```python
from build123d import *

# Parameters (mm, degrees)
SKETCH3_R           = 3.5
BOSS_EXTRUDE1_DEPTH = 304.8


with BuildPart() as part:
    # Sketch3 → Boss-Extrude1 (new, symmetric)
    with BuildSketch(Plane.XY):
        with BuildLine():
            Line((15.25, 20), (-15.25, 20))
            ThreePointArc((-15.25, 20), (-15.780330086, 19.780330086), (-16, 19.25))
            Line((-16, 19.25), (-16, 16.25))
            ThreePointArc((-16, 16.25), (-15.780330086, 15.719669914), (-15.25, 15.5))
            Line((-15.25, 15.5), (-9.931980515, 15.5))
            ThreePointArc((-9.931980515, 15.5), (-9.070942793, 14.924672987), (-9.272970773, 13.909009742))
            Line((-9.272970773, 13.909009742), (-15.140128061, 8.041852455))
            ThreePointArc((-15.140128061, 8.041852455), (-15.740311256, 7.640822865), (-16.448275606, 7.5))
            Line((-16.448275606, 7.5), (-23.551724394, 7.5))
            ThreePointArc((-23.551724394, 7.5), (-24.259688744, 7.640822865), (-24.859871939, 8.041852455))
            Line((-24.859871939, 8.041852455), (-30.727029227, 13.909009742))
            ThreePointArc((-30.727029227, 13.909009742), (-30.929057207, 14.924672987), (-30.068019485, 15.5))
            Line((-30.068019485, 15.5), (-24.75, 15.5))
            ThreePointArc((-24.75, 15.5), (-24.219669914, 15.719669914), (-24, 16.25))
            Line((-24, 16.25), (-24, 19.25))
            ThreePointArc((-24, 19.25), (-24.219669914, 19.780330086), (-24.75, 20))
            Line((-24.75, 20), (-37, 20))
            ThreePointArc((-37, 20), (-39.121320344, 19.121320344), (-40, 17))
            Line((-40, 17), (-40, 4.75))
            ThreePointArc((-40, 4.75), (-39.780330086, 4.219669914), (-39.25, 4))
            Line((-39.25, 4), (-36.25, 4))
            ThreePointArc((-36.25, 4), (-35.719669914, 4.219669914), (-35.5, 4.75))
            Line((-35.5, 4.75), (-35.5, 10.068019485))
            ThreePointArc((-35.5, 10.068019485), (-34.924672987, 10.929057207), (-33.909009742, 10.727029227))
            Line((-33.909009742, 10.727029227), (-28.041852455, 4.859871939))
            ThreePointArc((-28.041852455, 4.859871939), (-27.640822865, 4.259688744), (-27.5, 3.551724394))
            Line((-27.5, 3.551724394), (-27.5, -3.551724394))
            ThreePointArc((-27.5, -3.551724394), (-27.640822865, -4.259688744), (-28.041852455, -4.859871939))
            Line((-28.041852455, -4.859871939), (-33.909009742, -10.727029227))
            ThreePointArc((-33.909009742, -10.727029227), (-34.924672987, -10.929057207), (-35.5, -10.068019485))
            Line((-35.5, -10.068019485), (-35.5, -4.75))
            ThreePointArc((-35.5, -4.75), (-35.719669914, -4.219669914), (-36.25, -4))
            Line((-36.25, -4), (-39.25, -4))
            ThreePointArc((-39.25, -4), (-39.780330086, -4.219669914), (-40, -4.75))
            Line((-40, -4.75), (-40, -17))
            ThreePointArc((-40, -17), (-39.121320344, -19.121320344), (-37, -20))
            Line((-37, -20), (-24.75, -20))
            ThreePointArc((-24.75, -20), (-24.219669914, -19.780330086), (-24, -19.25))
            Line((-24, -19.25), (-24, -16.25))
            ThreePointArc((-24, -16.25), (-24.219669914, -15.719669914), (-24.75, -15.5))
            Line((-24.75, -15.5), (-30.068019485, -15.5))
            ThreePointArc((-30.068019485, -15.5), (-30.929057207, -14.924672987), (-30.727029227, -13.909009742))
            Line((-30.727029227, -13.909009742), (-24.859871939, -8.041852455))
            ThreePointArc((-24.859871939, -8.041852455), (-24.259688744, -7.640822865), (-23.551724394, -7.5))
            Line((-23.551724394, -7.5), (-16.448275606, -7.5))
            ThreePointArc((-16.448275606, -7.5), (-15.740311256, -7.640822865), (-15.140128061, -8.041852455))
            Line((-15.140128061, -8.041852455), (-9.272970773, -13.909009742))
            ThreePointArc((-9.272970773, -13.909009742), (-9.070942793, -14.924672987), (-9.931980515, -15.5))
            Line((-9.931980515, -15.5), (-15.25, -15.5))
            ThreePointArc((-15.25, -15.5), (-15.780330086, -15.719669914), (-16, -16.25))
            Line((-16, -16.25), (-16, -19.25))
            ThreePointArc((-16, -19.25), (-15.780330086, -19.780330086), (-15.25, -20))
            Line((-15.25, -20), (15.25, -20))
            ThreePointArc((15.25, -20), (15.780330086, -19.780330086), (16, -19.25))
            Line((16, -19.25), (16, -16.25))
            ThreePointArc((16, -16.25), (15.780330086, -15.719669914), (15.25, -15.5))
            Line((15.25, -15.5), (9.931980515, -15.5))
            ThreePointArc((9.931980515, -15.5), (9.070942793, -14.924672987), (9.272970773, -13.909009742))
            Line((9.272970773, -13.909009742), (15.140128061, -8.041852455))
            ThreePointArc((15.140128061, -8.041852455), (15.740311256, -7.640822865), (16.448275606, -7.5))
            Line((16.448275606, -7.5), (23.551724394, -7.5))
            ThreePointArc((23.551724394, -7.5), (24.259688744, -7.640822865), (24.859871939, -8.041852455))
            Line((24.859871939, -8.041852455), (30.727029227, -13.909009742))
            ThreePointArc((30.727029227, -13.909009742), (30.929057207, -14.924672987), (30.068019485, -15.5))
            Line((30.068019485, -15.5), (24.75, -15.5))
            ThreePointArc((24.75, -15.5), (24.219669914, -15.719669914), (24, -16.25))
            Line((24, -16.25), (24, -19.25))
            ThreePointArc((24, -19.25), (24.219669914, -19.780330086), (24.75, -20))
            Line((24.75, -20), (37, -20))
            ThreePointArc((37, -20), (39.121320344, -19.121320344), (40, -17))
            Line((40, -17), (40, -4.75))
            ThreePointArc((40, -4.75), (39.780330086, -4.219669914), (39.25, -4))
            Line((39.25, -4), (36.25, -4))
            ThreePointArc((36.25, -4), (35.719669914, -4.219669914), (35.5, -4.75))
            Line((35.5, -4.75), (35.5, -10.068019485))
            ThreePointArc((35.5, -10.068019485), (34.924672987, -10.929057207), (33.909009742, -10.727029227))
            Line((33.909009742, -10.727029227), (28.041852455, -4.859871939))
            ThreePointArc((28.041852455, -4.859871939), (27.640822865, -4.259688744), (27.5, -3.551724394))
            Line((27.5, -3.551724394), (27.5, 3.551724394))
            ThreePointArc((27.5, 3.551724394), (27.640822865, 4.259688744), (28.041852455, 4.859871939))
            Line((28.041852455, 4.859871939), (33.909009742, 10.727029227))
            ThreePointArc((33.909009742, 10.727029227), (34.924672987, 10.929057207), (35.5, 10.068019485))
            Line((35.5, 10.068019485), (35.5, 4.75))
            ThreePointArc((35.5, 4.75), (35.719669914, 4.219669914), (36.25, 4))
            Line((36.25, 4), (39.25, 4))
            ThreePointArc((39.25, 4), (39.780330086, 4.219669914), (40, 4.75))
            Line((40, 4.75), (40, 17))
            ThreePointArc((40, 17), (39.121320344, 19.121320344), (37, 20))
            Line((37, 20), (24.75, 20))
            ThreePointArc((24.75, 20), (24.219669914, 19.780330086), (24, 19.25))
            Line((24, 19.25), (24, 16.25))
            ThreePointArc((24, 16.25), (24.219669914, 15.719669914), (24.75, 15.5))
            Line((24.75, 15.5), (30.068019485, 15.5))
            ThreePointArc((30.068019485, 15.5), (30.929057207, 14.924672987), (30.727029227, 13.909009742))
            Line((30.727029227, 13.909009742), (24.859871939, 8.041852455))
            ThreePointArc((24.859871939, 8.041852455), (24.259688744, 7.640822865), (23.551724394, 7.5))
            Line((23.551724394, 7.5), (16.448275606, 7.5))
            ThreePointArc((16.448275606, 7.5), (15.740311256, 7.640822865), (15.140128061, 8.041852455))
            Line((15.140128061, 8.041852455), (9.272970773, 13.909009742))
            ThreePointArc((9.272970773, 13.909009742), (9.070942793, 14.924672987), (9.931980515, 15.5))
            Line((9.931980515, 15.5), (15.25, 15.5))
            ThreePointArc((15.25, 15.5), (15.780330086, 15.719669914), (16, 16.25))
            Line((16, 16.25), (16, 19.25))
            ThreePointArc((16, 19.25), (15.780330086, 19.780330086), (15.25, 20))
        make_face()
        with Locations(Location((-20, 0, 0), (0, 0, 180))):
            Circle(SKETCH3_R, mode=Mode.SUBTRACT)
        with Locations(Location((20, 0, 0), (0, 0, 180))):
            Circle(SKETCH3_R, mode=Mode.SUBTRACT)
        with BuildLine():
            Line((-2.25, -14.568019485), (-11.958147545, -4.859871939))
            ThreePointArc((-11.958147545, -4.859871939), (-12.359177135, -4.259688744), (-12.5, -3.551724394))
            Line((-12.5, -3.551724394), (-12.5, 3.551724394))
            ThreePointArc((-12.5, 3.551724394), (-12.359177135, 4.259688744), (-11.958147545, 4.859871939))
            Line((-11.958147545, 4.859871939), (-2.25, 14.568019485))
            ThreePointArc((-2.25, 14.568019485), (0, 15.5), (2.25, 14.568019485))
            Line((2.25, 14.568019485), (11.958147545, 4.859871939))
            ThreePointArc((11.958147545, 4.859871939), (12.359177135, 4.259688744), (12.5, 3.551724394))
            Line((12.5, 3.551724394), (12.5, -3.551724394))
            ThreePointArc((12.5, -3.551724394), (12.359177135, -4.259688744), (11.958147545, -4.859871939))
            Line((11.958147545, -4.859871939), (2.25, -14.568019485))
            ThreePointArc((2.25, -14.568019485), (0, -15.5), (-2.25, -14.568019485))
        make_face(mode=Mode.SUBTRACT)
    extrude(amount=BOSS_EXTRUDE1_DEPTH, both=True)


solid = part.part
```
Part model, mm, in its own coordinate system. A direction names the side the tool comes from. Round coordinates to 2 decimals unless told otherwise and drop trailing zeros. Answer as CSV lines item,"result". Start each with the question number.
1) Drop flat-ended pins along their axis: pin 1 (3 mm diameter, centred on y = -3.5, z = 174.5, fed in from +X); pin 2 (5.5 mm diameter, centred on x = -20, y = 0, fed in from +Z); pin 3 (0.9 mm diameter, centred on y = -18, z = -55, fed in from -X). Give the stop position or say it passes through.
2) Band-saw the part on A-A (z = -217). Count the separate pieces of the cut face and the enclosed holes in it, then the cut area to 3 significant figures.
3) Which spindle directions (+Z, -Z, +X, -X, +Y, -Y) get a long thin tool onto all of the face, cutting with end or side? Do faces 5 (the face through (7.17, -9.65, 4.27)), 6 (the face through (-31, 20, 4)). Say none if no direction does.
4) Drill centre lines: L1, parallel to X at y = -14.5, z = -169.5; L2, parallel to X at y = -17, z = -221; L3, parallel to Y at x = 26, z = -215. Where is each one in solid material? Low to high.
5) Mould opens along X. For faces 1 (the face through (-40, 11, 4)), 2 (the face through (-7.17, 9.65, 4.27)), 3 (the face through (7.04, 9.78, 4.27)), 4 (the face through (40, -11, 4)) say: +X half, -X half, draft (parallel to the pull), parting line (faces both ways), or undercut.
Worked out:
1,pin 1,"x = 40"
1,pin 2,"through"
1,pin 3,"x = -39.95"
2,separate pieces,"1"
2,enclosed holes,"3"
2,area,"1,590 mm²"
3,face 5,"+Z, -Z"
3,face 6,"+Z, -Z, +X, -X, +Y"
4,L1,"-40 to -31, -9 to -2.32, 2.32 to 9, 31 to 40"
4,L2,"-40 to -24, -16 to 16, 24 to 40"
4,L3,"-20 to -15.5, -9.18 to 9.18, 15.5 to 20"
5,face 1,"-X half"
5,face 2,"undercut"
5,face 3,"undercut"
5,face 4,"+X half"
